Could you check a few things on this drawing? It's one solid part, dimensions in mm from its lowest x, y, z. A direction names the side the tool comes from. Give positions to 0.01 mm unless a question says otherwise; leave off trailing zeros. Write each loop counter-clockwise with the first axis right and the second up, starting at its lowest first coordinate (ties: lowest second). Pieces come first, ordered by that corner, then holes. Notation, with made-up numbers: (40.25, 18) - (70.25, 18) arc R18 cw to (70.25, 36) - close; hole circle Ø6 at (10.5, -18). An arc over 180 degrees is marked (long way). One line per item, written item: value. Start each with the question number.
1) On a 3-axis mill with a long thin cutter (end or side, diameter ignored), from which of +Z, -Z, +X, -X, +Y, -Y can I reach the whole of each face in a straight line? I mean the marked faces 5 and 6. Say none if no direction works.
2) We'd pull the mould along Z, two halves only. Please class the marked faces 1, 2, 3 and 4: +Z half, -Z half, draft (parallel to the pull), parting line (faces both ways), or undercut.
3) Imagine slicing it at A-A on y = 38. Write out the boundary of the cut face in (x, z), plus the area to 3 significant figures.
4) Imagine slicing it at B-B on x = 39.5. Write out the boundary of the cut face in (y, z).
5) Please list where these lines run through material, in increasing order: L1, parallel to Y at x = 17, z = 57; L2, parallel to Z at x = 39, y = 84; L3, parallel to Y at x = 28, z = 30. Write a range as [from, to].
6) Imagine slicing it at C-C on z = 84.3. Write out the boundary of the cut face in (x, y), plus the area to 3 significant figures.
7) I'm going to push flat-ended pins straight in: P1, Ø1, axis at y = 26, z = 70, coming from the -X side; P2, Ø3.5, axis at y = 12.7, z = 57.15, coming from the -X side. Where does each tip first touch, or does it pass through?
8) Imagine slicing it at D-D on x = 6.5. Write out the boundary of the cut face in (y, z), plus the area to 3 significant figures.
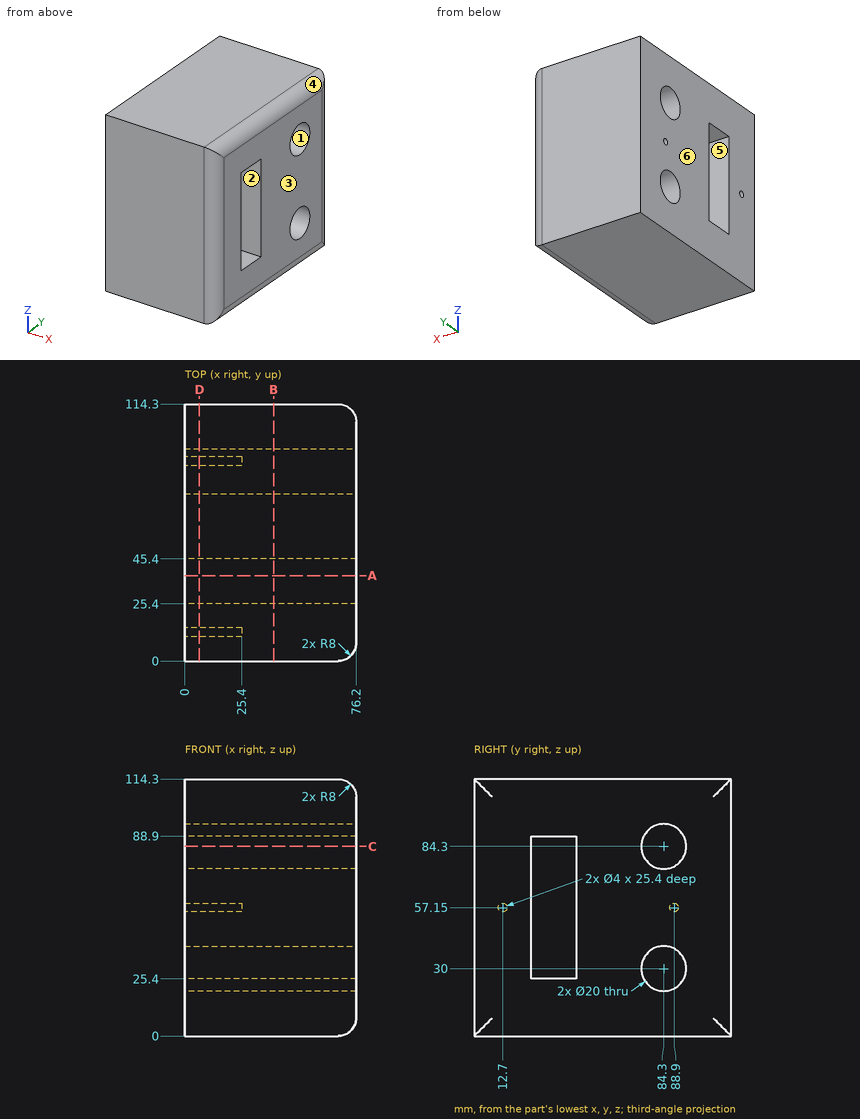
Numbers:
1. face 5: +X, -X
1. face 6: +Z, -Z, -X, +Y, -Y
2. face 1: undercut
2. face 2: undercut
2. face 3: draft
2. face 4: +Z half
3. outline: (0, 0) - (68.2, 0) arc R8 ccw to (76.2, 8) - (76.2, 25.4) - (0, 25.4) - close; (0, 88.9) - (76.2, 88.9) - (76.2, 106.3) arc R8 ccw to (68.2, 114.3) - (0, 114.3) - close
3. area: 3,840 mm^2
4. outline: (0, 0) - (114.3, 0) - (114.3, 114.3) - (0, 114.3) - close; hole (25.4, 25.4) - (45.4, 25.4) - (45.4, 88.9) - (25.4, 88.9) - close; hole circle Ø20 at (84.3, 30); hole circle Ø20 at (84.3, 84.3)
5. L1: [0, 10.71], [14.69, 25.4], [45.4, 86.91], [90.89, 114.3]
5. L2: [0, 20], [40, 74.3], [94.3, 114.3]
5. L3: [0, 25.4], [45.4, 74.3], [94.3, 114.3]
6. outline: (0, 0) - (68.2, 0) arc R8 ccw to (76.2, 8) - (76.2, 25.4) - (0, 25.4) - close; (0, 45.4) - (76.2, 45.4) - (76.2, 74.3) - (0, 74.3) - close; (0, 94.3) - (76.2, 94.3) - (76.2, 106.3) arc R8 ccw to (68.2, 114.3) - (0, 114.3) - close
6. area: 5,630 mm^2
7. P1: through
7. P2: x = 25.4
8. outline: (0, 0) - (114.3, 0) - (114.3, 114.3) - (0, 114.3) - close; hole circle Ø4 at (12.7, 57.15); hole (25.4, 25.4) - (45.4, 25.4) - (45.4, 88.9) - (25.4, 88.9) - close; hole circle Ø20 at (84.3, 30); hole circle Ø20 at (84.3, 84.3); hole circle Ø4 at (88.9, 57.15)
8. area: 11,100 mm^2
